```python
from build123d import *

# Parameters (mm, degrees)
SKETCH_1_W          = 100
SKETCH_1_H          = 76
EXTRUDE_1_DEPTH     = 12
SKETCH_2_W          = 97
SKETCH_2_H          = 73
CUT_EXTRUDE_1_DEPTH = 10
SKETCH_3_R          = 1.65
CUT_EXTRUDE_2_DEPTH = 127.174482365


with BuildPart() as part:
    # 草图1 → 凸台-拉伸1 (new body)
    with BuildSketch(Plane(origin=(0, 0, 0), x_dir=(1, 0, 0), z_dir=(0, 1, 0))):
        with Locations((50, 38)):
            Rectangle(SKETCH_1_W, SKETCH_1_H)
    extrude(amount=EXTRUDE_1_DEPTH)

    # 草图2 → 切除-拉伸1 (cut)
    with BuildSketch(Plane(origin=(0, 12, 0), x_dir=(1, 0, 0), z_dir=(0, 1, 0))):
        with Locations((50, 38)):
            Rectangle(SKETCH_2_W, SKETCH_2_H)
    extrude(amount=-CUT_EXTRUDE_1_DEPTH, mode=Mode.SUBTRACT)

    # 草图3 → 切除-拉伸2 (cut, through all)
    with BuildSketch(Plane(origin=(0, 0, -76), x_dir=(-1, 0, 0), z_dir=(0, 0, -1))):
        with Locations((-90, 6)):
            Circle(SKETCH_3_R)
        with Locations((-10, 6)):
            Circle(SKETCH_3_R)
        with Locations((-50, 6)):
            Circle(SKETCH_3_R)
    extrude(amount=-CUT_EXTRUDE_2_DEPTH, mode=Mode.SUBTRACT)


solid = part.part
```
The listing builds one solid part. Answer for the finished solid, in the listing's coordinates (mm). A direction names the side the tool comes from. Coordinates: 2 decimals unless noted, no trailing zeros. Loops run counter-clockwise (first coordinate to the right, second up) from the corner with the lowest first, then second, coordinate; pieces in that order, holes last. Notation, with made-up numbers: (84, 21.5) -> (100, 21.5) arc R14 cw to (100, 42.5) -> close; hole circle Ø10 at (43.25, -9.5). An arc over 180 degrees is marked (long way). Return JSON: item names as keys, results as strings. Group by question number.
(1) Given pin 1 Ø5 at (x, z) = (77, -21.5) entering from +Y, flat-ended and moving along its own axis, determine where the tip first touches the part or whether it passes through.
(2) A cutting plane is placed at D-D on x = 23. Write down the section's boundary in (y, z).
(3) Find the intervals of material crossed by probe 1 along Y at (x, z) = (90, -0.4); probe 2 along Z at (x, y) = (8.5, 8); probe 3 along X at (y, z) = (10, -23.5), in increasing order. Write a range as from..to.
(4) A cutting plane is placed at B-B on x = 10. Write down the section's boundary in (y, z).
(5) A cutting plane is placed at C-C on z = -69. Write down the section's boundary in (x, y).
(6) Determine the mould class of faces 3 (the flat face through (49, 2, -39)), 4 (the flat face through (49, 3, 0)), 5 (the flat face through (49, 8, -1.5)), 6 (the cylindrical face through (50.4, 4.4, -0.8)) for opening direction Z: released by +Z, released by -Z, zero draft, split by the parting line, or undercut.
(7) A cutting plane is placed at A-A on y = 6. Count the separate pieces of the cut face and the enclosed holes in it, and give its area (3 significant figures).
(8) Which of the six approach directions +Z, -Z, +X, -X, +Y, -Y give full straight-line access (tool end or side, diameter ignored) to faces 1 (the flat face through (1.5, 7, -37)), 2 (the flat face through (100, 6, -37))?
The answers:
{
 "1": {"pin 1": "stops at y = 2"},
 "2": {"outline": "(0, -76) -> (12, -76) -> (12, -74.5) -> (2, -74.5) -> (2, -1.5) -> (12, -1.5) -> (12, 0) -> (0, 0) -> close"},
 "3": {"probe 1": "y = 0..4.35, 7.65..12", "probe 2": "z = -76..-74.5, -1.5..0", "probe 3": "x = 0..1.5, 98.5..100"},
 "4": {"outline": "(0, -76) -> (4.35, -76) -> (4.35, -74.5) -> (2, -74.5) -> (2, -1.5) -> (4.35, -1.5) -> (4.35, 0) -> (0, 0) -> close; (7.65, -76) -> (12, -76) -> (12, -74.5) -> (7.65, -74.5) -> close; (7.65, -1.5) -> (12, -1.5) -> (12, 0) -> (7.65, 0) -> close"},
 "5": {"outline": "(0, 0) -> (100, 0) -> (100, 12) -> (98.5, 12) -> (98.5, 2) -> (1.5, 2) -> (1.5, 12) -> (0, 12) -> close"},
 "6": {"face 3": "undercut", "face 4": "released by +Z", "face 5": "undercut", "face 6": "zero draft"},
 "7": {"separate pieces": "6", "enclosed holes": "0", "area": "489 mm^2"},
 "8": {"face 1": "+Y", "face 2": "+Z, -Z, +X, +Y, -Y"}
}
